The model under review builds one solid part; all positions refer to its coordinate system, in mm. A direction names the side the tool comes from. Round coordinates to 2 decimals unless told otherwise and drop trailing zeros. Return JSON: item names as keys, results as strings. Group by question number.
Q1. Draft analysis for pull direction X (two halves, no side actions). For faces 1 (the face through (-160, -40, -84)), 2 (the face through (76.668, -0.952, -67.984)), 3 (the face through (142.15, -18.01, -83.81)), state which applies: pulls with the +X half, pulls with the -X half, needs draft (parallel to the pull), parting line crosses it, or undercut.
Q2. For faces 4 (the face through (94.05, -18.01, -83.81)), 5 (the face through (155, 0, -84)), 6 (the face through (-190, 36, -84)), 7 (the face through (0.5, 88, -86)), list the 3-axis set-ups (+Z, -Z, +X, -X, +Y, -Y) from which the entire face can be reached by the end or side of a thin tool; tool diameter is ignored.
Q3. Consider section A-A (z = -60). Count the separate pieces of the cut face and the enclosed holes in it, and give its area (3 significant figures).
Q4. To check wall thickness, follow line 1 along Z through (x, y) = (-56.5, -2); line 2 along X through (y, z) = (-30.5, -73.5); line 3 along X through (y, z) = (20, -39). State the ranges of each line that lie inside material, in increasing order.
Q5. Clearance check with flat-ended pins moving along their axes: pin 1 Ø18.5 at (y, z) = (-2, -60) entering from -X; pin 2 Ø8 at (x, z) = (143.5, -19) entering from -Y; pin 3 Ø4 at (x, z) = (79, -62.5) entering from -Y. State where each tip first meets the part, or that it passes through.
from build123d import *

# Parameters (mm, degrees)
SKETCH1_RX              = 240
SKETCH1_RY              = 110
BOSS_EXTRUDE1_DEPTH     = 170
SKETCH9_W               = 85
SKETCH9_H               = 81
CUT_EXTRUDE4_DEPTH      = 315.006369362
CUT_EXTRUDE5_DEPTH      = 305.024031405
CUT_EXTRUDE6_DEPTH      = 305.024031405
CUT_EXTRUDE6_DEPTH_BACK = 305.024031405
SKETCH11_R              = 8.05220018
SKETCH11_R_2            = 2.75
CHAMFER1_START          = -171
CHAMFER1_DEPTH          = 172
CUT_EXTRUDE7_DEPTH      = 302.762319701
CHAMFER2_SIZE           = 10
CUT_EXTRUDE8_DEPTH      = 302.762319701
CUT_EXTRUDE8_DEPTH_BACK = 302.762319701
SKETCH14_W              = 1
SKETCH14_H              = 125
CUT_EXTRUDE9_DEPTH      = 302.762319832
CUT_EXTRUDE9_DEPTH_BACK = 302.762319832
FILLET1_R               = 10
FILLET2_R               = 3
CHAMFER4_SIZE           = 10


with BuildPart() as part:
    # Sketch1 → Boss-Extrude1 (new body)
    with BuildSketch(Plane.XY):
        with Locations((0, 0)):
            Ellipse(SKETCH1_RX, SKETCH1_RY)
    extrude(amount=-BOSS_EXTRUDE1_DEPTH)

    # Sketch9 → Cut-Extrude4 (cut, through all)
    with BuildSketch(Plane.XY):
        with Locations((197.5, -4.5)):
            Rectangle(SKETCH9_W, SKETCH9_H)
        with Locations((-197.5, -4.5)):
            Rectangle(SKETCH9_W, SKETCH9_H)
    extrude(amount=-CUT_EXTRUDE4_DEPTH, mode=Mode.SUBTRACT)

    # Sketch10 → Cut-Extrude5 (cut, through all)
    with BuildSketch(Plane.XY):
        Polygon((-137.5, 83.1), (137.5, 83.1), (137.5, 28.1), (142.5, 28.1), (142.5, 25.1), (137.5, 25.1), (137.5, 15.1), (-137.5, 15.1), (-137.5, 25.1), (-142.5, 25.1), (-142.5, 28.1), (-137.5, 28.1), align=None)
    extrude(amount=-CUT_EXTRUDE5_DEPTH, mode=Mode.SUBTRACT)

    # Sketch11 → Cut-Extrude6 (cut, two sides: drawn at the far end of the back side and taken through both)
    with BuildSketch(Plane(origin=(0, 0, 0), x_dir=(0, 0, -1), z_dir=(1, 0, 0)).offset(-CUT_EXTRUDE6_DEPTH_BACK)):
        with Locations(Location((60, -2, 0), (0, 0, 270))):
            Circle(SKETCH11_R)
        with Locations(Location((150, -2, 0), (0, 0, 270))):
            Circle(SKETCH11_R_2)
    extrude(amount=CUT_EXTRUDE6_DEPTH + CUT_EXTRUDE6_DEPTH_BACK, mode=Mode.SUBTRACT)

    # Chamfer1: read off the stored shape, not the designer's step
    # Chamfer1 outline → Chamfer1 (cut)
    with BuildSketch(Plane.XY.offset(CHAMFER1_START)):
        with BuildLine():
            add(Edge.make_bspline(
                [(226.783181851, 36), (225.338784139, 37.911428345), (223.742033582, 39.797224556)],
                knots=[0.33341591, 0.33341591, 0.33341591, 0.380954959, 0.380954959, 0.380954959], degree=2, weights=[1, 0.98707721, 0.974650902]))
            Line((223.742033582, 39.797224556), (223.213573476, 36))
            Line((223.213573476, 36), (226.783181851, 36))
        make_face()
        with BuildLine():
            Line((-223.213573476, 36), (-223.742033582, 39.797224556))
            add(Edge.make_bspline(
                [(-223.742033582, 39.797224556), (-225.338784139, 37.911428345), (-226.783181851, 36)],
                knots=[2.760637694, 2.760637694, 2.760637694, 2.808176743, 2.808176743, 2.808176743], degree=2, weights=[0.974650902, 0.98707721, 1]))
            Line((-226.783181851, 36), (-223.213573476, 36))
        make_face()
        with BuildLine():
            add(Edge.make_bspline(
                [(-218.998471635, -45), (-217.313455553, -46.722643886), (-215.500461662, -48.417772396)],
                knots=[3.563050222, 3.563050222, 3.563050222, 3.605808591, 3.605808591, 3.605808591], degree=2, weights=[1, 0.989008328, 0.978425575]))
            Line((-215.500461662, -48.417772396), (-215.462722195, -45))
            Line((-215.462722195, -45), (-218.998471635, -45))
        make_face()
        with BuildLine():
            Line((215.462722195, -45), (215.500461662, -48.417772396))
            add(Edge.make_bspline(
                [(215.500461662, -48.417772396), (217.313455553, -46.722643886), (218.998471635, -45)],
                knots=[5.818969369, 5.818969369, 5.818969369, 5.861727739, 5.861727739, 5.861727739], degree=2, weights=[0.978425575, 0.989008328, 1]))
            Line((218.998471635, -45), (215.462722195, -45))
        make_face()
    extrude(amount=CHAMFER1_DEPTH, mode=Mode.SUBTRACT)

    # Sketch13 → Cut-Extrude7 (cut, through all)
    with BuildSketch(Plane.XY):
        Polygon((-76.2, -81.5), (-76.2, -93.9), (76.2, -93.9), (76.2, -81.5), (81.2, -81.5), (81.2, -78.5), (76.2, -78.5), (76.2, -15), (-76.2, -15), (-76.2, -78.5), (-81.2, -78.5), (-81.2, -81.5), align=None)
    extrude(amount=-CUT_EXTRUDE7_DEPTH, mode=Mode.SUBTRACT)

    # Chamfer2
    chamfer2_edges = [part.edges().sort_by_distance(p)[0] for p in [
        (155, -45, -85),
        (-155, -45, -85),
    ]]
    chamfer(chamfer2_edges, length=CHAMFER2_SIZE)

    # Sketch14 → Cut-Extrude8 (cut, two sides: drawn at the far end of the back side and taken through both)
    with BuildSketch(Plane.XY.offset(-CUT_EXTRUDE8_DEPTH_BACK)):
        with Locations((0, 47.5)):
            Rectangle(SKETCH14_W, SKETCH14_H)
    extrude(amount=CUT_EXTRUDE8_DEPTH + CUT_EXTRUDE8_DEPTH_BACK, mode=Mode.SUBTRACT)

    # Sketch15 → Cut-Extrude9 (cut, two sides: drawn at the far end of the back side and taken through both)
    with BuildSketch(Plane.XY.offset(-CUT_EXTRUDE9_DEPTH_BACK)):
        with BuildLine():
            Line((147.5, 75.514694834), (147.5, 46))
            Line((147.5, 46), (199.781755924, 46))
            add(Edge.make_bspline(
                [(199.781755924, 46), (179.990233789, 62.979001801), (147.5, 75.514694834)],
                knots=[3.619587852, 3.619587852, 3.619587852, 3.997470903, 3.997470903, 3.997470903], degree=2, weights=[1, 0.982203587, 1]))
        make_face()
        with BuildLine():
            Line((91.2, -91.41689608), (91.2, -15))
            Line((91.2, -15), (145, -15))
            Line((145, -15), (145, -76.465113485))
            add(Edge.make_bspline(
                [(91.2, -91.41689608), (120.495747781, -85.643811522), (145, -76.465113485)],
                knots=[1.988139758, 1.988139758, 1.988139758, 2.27109284, 2.27109284, 2.27109284], degree=2, weights=[1, 0.990008876, 1]))
        make_face()
        with BuildLine():
            Line((-82.129314955, 93.1), (82.129314955, 93.1))
            add(Edge.make_bspline(
                [(82.129314955, 93.1), (0, 107.411385607), (-82.129314955, 93.1)],
                knots=[4.338735578, 4.338735578, 4.338735578, 5.086042382, 5.086042382, 5.086042382], degree=2, weights=[1, 0.931, 1]))
        make_face()
        with BuildLine():
            Line((-91.2, -91.41689608), (-91.2, -15))
            Line((-91.2, -15), (-145, -15))
            Line((-145, -15), (-145, -76.465113485))
            add(Edge.make_bspline(
                [(-145, -76.465113485), (-120.495747781, -85.643811522), (-91.2, -91.41689608)],
                knots=[0.870499814, 0.870499814, 0.870499814, 1.153452896, 1.153452896, 1.153452896], degree=2, weights=[1, 0.990008876, 1]))
        make_face()
        with BuildLine():
            Line((-147.5, 75.514694834), (-147.5, 46))
            Line((-147.5, 46), (-199.781755924, 46))
            add(Edge.make_bspline(
                [(-147.5, 75.514694834), (-179.990233789, 62.979001801), (-199.781755924, 46)],
                knots=[5.427307058, 5.427307058, 5.427307058, 5.805190109, 5.805190109, 5.805190109], degree=2, weights=[1, 0.982203587, 1]))
        make_face()
    extrude(amount=CUT_EXTRUDE9_DEPTH + CUT_EXTRUDE9_DEPTH_BACK, mode=Mode.SUBTRACT)

    # Fillet1
    fillet1_edges = [part.edges().sort_by_distance(p)[0] for p in [
        (-145, -15, -85),
        (-145, -76.465113485, -85),
        (-91.2, -91.41689608, -85),
        (145, -76.465113485, -85),
        (91.2, -91.41689608, -85),
        (91.2, -15, -85),
        (-91.2, -15, -85),
        (145, -15, -85),
    ]]
    fillet(fillet1_edges, radius=FILLET1_R)

    # Fillet2
    fillet2_edges = [part.edges().sort_by_distance(p)[0] for p in [
        (-82.129314955, 93.1, -85),
        (82.129314955, 93.1, -85),
        (199.781755924, 46, -85),
        (147.5, 75.514694834, -85),
        (147.5, 46, -85),
        (-147.5, 75.514694834, -85),
        (-147.5, 46, -85),
        (-199.781755924, 46, -85),
    ]]
    fillet(fillet2_edges, radius=FILLET2_R)

    # Chamfer4
    chamfer4_edges = [part.edges().sort_by_distance(p)[0] for p in [
        (-137.5, 83.1, -85),
        (137.5, 83.1, -85),
    ]]
    chamfer(chamfer4_edges, length=CHAMFER4_SIZE)


solid = part.part
Values:
{
 "1": {"face 1": "pulls with the -X half", "face 2": "needs draft", "face 3": "undercut"},
 "2": {"face 4": "+Z, -Z", "face 5": "+Z, -Z, +X", "face 6": "+Z, -Z, -X", "face 7": "+Z, -Z, +Y"},
 "3": {"separate pieces": "3", "enclosed holes": "4", "area": "25,000 mm2"},
 "4": {"line 1": "z = -170 to -152.75, -147.25 to -68.05, -51.95 to 0", "line 2": "x = -155 to -145, -91.2 to -76.2, 76.2 to 91.2, 145 to 155", "line 3": "x = -155 to -137.5, 137.5 to 155"},
 "5": {"pin 1": "stops at x = -155", "pin 2": "stops at y = -89.51", "pin 3": "stops at y = -104.18"}
}
